from build123d import *

# Parameters (mm, degrees)
ESBO_O1_W                = 250
ESBO_O1_H                = 120
RESSALTO_EXTRUS_O1_DEPTH = 100
ESBO_O2_W                = 112
ESBO_O2_H                = 50
CORTE_EXTRUS_O1_DEPTH    = 70
ESBO_O3_W                = 54
ESBO_O3_H                = 3
CORTE_EXTRUS_O2_DEPTH    = 118
ESBO_O5_W                = 112
ESBO_O5_H                = 185
CORTE_EXTRUS_O3_DEPTH    = 70
ESBO_O6_W                = 114
ESBO_O6_H                = 3
CORTE_EXTRUS_O4_DEPTH    = 192
ESBO_O7_W                = 114
ESBO_O7_H                = 26
CORTE_EXTRUS_O5_DEPTH    = 500
ESBO_O8_W                = 5
ESBO_O8_H                = 179
CORTE_EXTRUS_O6_DEPTH    = 500
ESBO_O9_W                = 29
ESBO_O9_H                = 26
CORTE_EXTRUS_O7_DEPTH    = 500
ESBO_O10_R               = 5.45
CORTE_EXTRUS_O8_DEPTH    = 10


with BuildPart() as part:
    # Esboço1 → Ressalto-extrusão1 (new body)
    with BuildSketch(Plane(origin=(0, 0, 0), x_dir=(0, 1, 0), z_dir=(0, 0, 1))):
        Rectangle(ESBO_O1_W, ESBO_O1_H)
    extrude(amount=RESSALTO_EXTRUS_O1_DEPTH)

    # Esboço2 → Corte-extrusão1 (cut)
    with BuildSketch(Plane.XY.offset(100)):
        with Locations((0, 96)):
            Rectangle(ESBO_O2_W, ESBO_O2_H)
    extrude(amount=-CORTE_EXTRUS_O1_DEPTH, mode=Mode.SUBTRACT)

    # Esboço3 → Corte-extrusão2 (cut)
    with BuildSketch(Plane(origin=(-60, 0, 0), x_dir=(0, -1, 0), z_dir=(-1, 0, 0))):
        with Locations((-96, 95.5)):
            Rectangle(ESBO_O3_W, ESBO_O3_H)
    extrude(amount=-CORTE_EXTRUS_O2_DEPTH, mode=Mode.SUBTRACT)

    # Esboço5 → Corte-extrusão3 (cut)
    with BuildSketch(Plane.XY.offset(100)):
        with Locations((0, -28.5)):
            Rectangle(ESBO_O5_W, ESBO_O5_H)
    extrude(amount=-CORTE_EXTRUS_O3_DEPTH, mode=Mode.SUBTRACT)

    # Esboço6 → Corte-extrusão4 (cut)
    with BuildSketch(Plane.XZ.offset(125)):
        with Locations((0, 95.5)):
            Rectangle(ESBO_O6_W, ESBO_O6_H)
    extrude(amount=-CORTE_EXTRUS_O4_DEPTH, mode=Mode.SUBTRACT)

    # Esboço7 → Corte-extrusão5 (cut)
    with BuildSketch(Plane.XZ.offset(125)):
        with Locations((0, 13)):
            Rectangle(ESBO_O7_W, ESBO_O7_H)
    extrude(amount=-CORTE_EXTRUS_O5_DEPTH, mode=Mode.SUBTRACT)

    # Esboço8 → Corte-extrusão6 (cut)
    with BuildSketch(Plane.XY.offset(30)):
        with Locations((-50.5, -28.5)):
            Rectangle(ESBO_O8_W, ESBO_O8_H)
    corte_extrus_o6 = extrude(amount=-CORTE_EXTRUS_O6_DEPTH, mode=Mode.SUBTRACT)

    # Espelhar1: Corte-extrusão6 across plane
    add(corte_extrus_o6.mirror(Plane(origin=(0, 0, 0), x_dir=(0, 0, 1), z_dir=(1, 0, 0))), mode=Mode.SUBTRACT)

    # Esboço9 → Corte-extrusão7 (cut)
    with BuildSketch(Plane(origin=(-60, 0, 0), x_dir=(0, -1, 0), z_dir=(-1, 0, 0))):
        with Locations((-95.5, 13)):
            Rectangle(ESBO_O9_W, ESBO_O9_H)
    corte_extrus_o7 = extrude(amount=-CORTE_EXTRUS_O7_DEPTH, mode=Mode.SUBTRACT)

    # Espelhar2: Corte-extrusão7 across plane
    add(corte_extrus_o7.mirror(Plane.ZX), mode=Mode.SUBTRACT)

    # Esboço10 → Corte-extrusão8 (cut)
    with BuildSketch(Plane.YZ.offset(60)):
        with Locations((95, 60)):
            Circle(ESBO_O10_R)
    extrude(amount=-CORTE_EXTRUS_O8_DEPTH, mode=Mode.SUBTRACT)


solid = part.part
Verification items for the finished model (mm, model axes). A direction names the side the tool comes from. Coordinates: 2 decimals unless noted, no trailing zeros. Order: outer loops, then holes, each group sorted by start corner. A loop starts at its lowest first (then second) coordinate and runs counter-clockwise, first axis right, second up. Notation, with made-up numbers: M -28,35.5 L 1,35.5 A23 cw 1,54.5 Z; hole C 70.5,47 d10. An arc over 180 degrees is marked long. One line per item, written item: value. Start each with the question number.
Item 1: Thickness scan on probe 1 along Y at (x, z) = (-42, 61.5); probe 2 along Z at (x, y) = (57.4, 95); probe 3 along X at (y, z) = (-113.5, 77). Record the ranges inside material, lowest first.
Item 2: Sectioned sample at C-C on x = -36. Record the cut outline in (y, z), then the cut area to 3 significant figures.
Item 3: Depth check by flat-ended pin: P1, Ø4, axis at x = 8.5, y = -65.5, coming from the +Z side; P2, Ø0.9, axis at y = 96, z = 95, coming from the -X side. Enter the tip coordinate at first touch or a pass-through.
Item 4: Sectioned sample at D-D on z = 60. Record the cut outline in (x, y), then the cut area to 3 significant figures.
Item 5: Mould release check, pull along Y, two halves, no side actions. Record for faces 1 (the flat face through (1, 125, 60)), 2 (the flat face through (-57, -118, 13)), 3 (the flat face through (-1, 71, 62)): pulls with the +Y half, pulls with the -Y half, needs draft (parallel to the pull), parting line crosses it, or undercut.
Item 6: Sectioned sample at B-B on z = 76. Record the cut outline in (x, y), then the cut area to 3 significant figures.
Item 7: Sectioned sample at A-A on y = -46.5. Record the cut outline in (x, z).
Item 8: Access from +Z, -Z, +X, -X, +Y, -Y to the whole of each face (thin tool, end or side, straight path). Record for faces 4 (the flat face through (0, -122, 94)), 5 (the cylindrical face through (58.028, 100.198, 61.637)), 6 (the flat face through (-19, 122, 97)), 7 (the flat face through (57, -118, 13)), 8 (the flat face through (-56, 96, 62)).
Calculated:
1. probe 1: -125 to -121, 64 to 71, 121 to 125
1. probe 2: 26 to 54.55, 65.45 to 94, 97 to 100
1. probe 3: -60 to -56, 56 to 60
2. outline: M -125,26 L 125,26 L 125,100 L 121,100 L 121,97 L 123,97 L 123,94 L 121,94 L 121,30 L 71,30 L 71,94 L 69,94 L 69,97 L 71,97 L 71,100 L 64,100 L 64,97 L 67,97 L 67,94 L 64,94 L 64,30 L -121,30 L -121,94 L -125,94 Z; M -125,97 L -121,97 L -121,100 L -125,100 Z
2. area: 2,020 mm^2
3. P1: z = 30
3. P2: x = 58
4. outline: M -60,-125 L 60,-125 L 60,89.55 L 56,89.55 L 56,71 L -56,71 L -56,121 L 56,121 L 56,100.45 L 60,100.45 L 60,125 L -60,125 Z; hole M -56,-121 L 56,-121 L 56,64 L -56,64 Z
4. area: 3,640 mm^2
5. face 1: pulls with the +Y half
5. face 2: needs draft
5. face 3: undercut
6. outline: M -60,-125 L 60,-125 L 60,125 L -60,125 Z; hole M -56,-121 L 56,-121 L 56,64 L -56,64 Z; hole M -56,71 L 56,71 L 56,121 L -56,121 Z
6. area: 3,680 mm^2
7. outline: M -60,0 L -57,0 L -57,26 L -53,26 L -53,30 L -56,30 L -56,94 L -57,94 L -57,97 L -56,97 L -56,100 L -60,100 Z; M -48,26 L 48,26 L 48,30 L -48,30 Z; M 53,26 L 57,26 L 57,0 L 60,0 L 60,100 L 56,100 L 56,97 L 57,97 L 57,94 L 56,94 L 56,30 L 53,30 Z
8. face 4: -Y
8. face 5: +X
8. face 6: -X
8. face 7: -Z, +Y, -Y
8. face 8: +Z
